Read the model definition and answer for the solid it produces. Units are mm, in the model's axes. Coordinates: 2 decimals unless noted, no trailing zeros. Loops run counter-clockwise (first coordinate to the right, second up) from the corner with the lowest first, then second, coordinate; pieces in that order, holes last.
Autodesk Inventor part; units mm, degrees
ref_plane "YZ Plane" through (0, 0, 0) normal (1, 0, 0) x (0, 1, 0)
ref_plane "XZ Plane" through (0, 0, 0) normal (0, 1, 0) x (-1, 0, 0)
ref_plane "XY Plane" through (0, 0, 0) normal (0, 0, 1) x (1, 0, 0)
sketch "Sketch1" plane through (0, 0, 0) normal (0, 0, 1) x (1, 0, 0)
  line L0 (3.6662, -6.35) -> (-3.6662, -6.35)
  line L1 (-3.6662, -6.35) -> (-7.3323, 0)
  line L2 (-7.3323, 0) -> (-3.6662, 6.35)
  line L3 (-3.6662, 6.35) -> (3.6662, 6.35)
  line L4 (3.6662, 6.35) -> (7.3323, 0)
  line L5 (7.3323, 0) -> (3.6662, -6.35)
  point P0 (0, 0)
  point P1 (0, 0)
  dimension "d0" = 12.7
extrude "Extrusion1" add sketch "Sketch1" along normal blind 61.8617
sketch "Sketch2" plane through (0, 0, 61.8617) normal (0, 0, 1) x (1, 0, 0)
  point P0 (0, 0)
  point P1 (0, 0)
hole "Hole1" at (0, 0, 61.8617) direction (0, 0, -1) diameter 3.9624 depth 13.6144 tip angle 118
sketch "Sketch3" plane through (0, 0, 0) normal (0, 0, -1) x (-1, 0, 0)
  circle A0 centre (0, 0) radius 1.9812
hole "Hole2" at (0, 0, 0) direction (0, 0, 1) diameter 3.9624 depth 13.6144 tip angle 118
properties part number "STOCK,HEX,SHAFT,TURRET,ENCODER" material "Aluminum 6061"
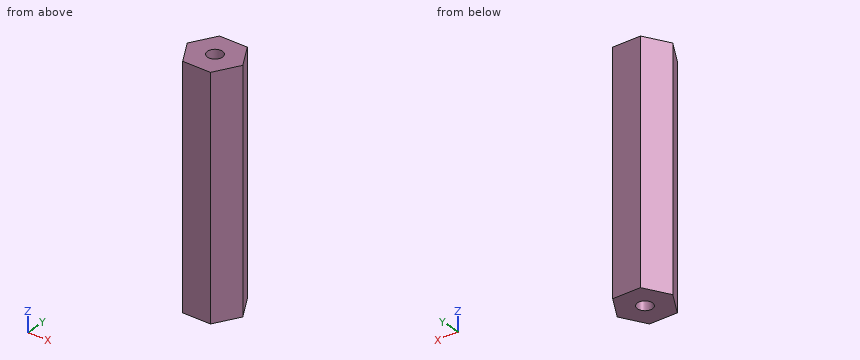
Q1. A cutting plane is placed at A-A (z = 38). Give the vertices of the cut face in (x, y), then the cut area to 3 significant figures.
Findings below:
outline: (-7.33, 0) - (-3.67, -6.35) - (3.67, -6.35) - (7.33, 0) - (3.67, 6.35) - (-3.67, 6.35) - close
area: 140 mm2
Q2. A flat-ended cylindrical pin translates along its axis: pin 1 Ø1 at (x, z) = (-5.5, 36) entering from +Y. Find the tip coordinate at first contact, or state that the pin passes through.
Findings below:
pin 1: stops at y = 4.04
Q3. A cutting plane is placed at C-C (y = 3). Give the vertices of the cut face in (x, z).
Findings below:
outline: (-5.6, 0) - (5.6, 0) - (5.6, 61.86) - (-5.6, 61.86) - close
Q4. A cutting plane is placed at B-B (x = 5). Give the vertices of the cut face in (y, z).
Findings below:
outline: (-4.04, 0) - (4.04, 0) - (4.04, 61.86) - (-4.04, 61.86) - close
Q5. Straight lines are drawn through the part: probe 1 along X at (y, z) = (0, 7); probe 2 along Y at (x, z) = (0, 7); probe 3 along Y at (x, z) = (-0.75, 50). For each, find the intervals that lie inside material, in ascending order.
Findings below:
probe 1: x = -7.33 to -1.98, 1.98 to 7.33
probe 2: y = -6.35 to -1.98, 1.98 to 6.35
probe 3: y = -6.35 to -1.83, 1.83 to 6.35
